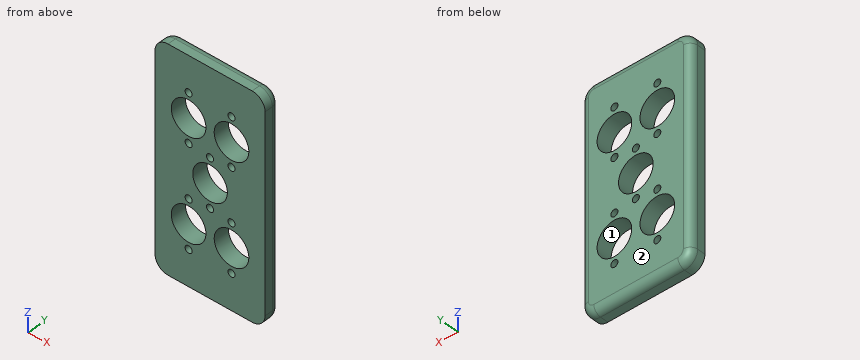
from build123d import *

# Parameters (mm, degrees)
SKETCH1_W             = 50.8
SKETCH1_H             = 101.6
BOSS_EXTRUDE1_DEPTH   = 7.25
FILLET1_R             = 6
FILLET2_R             = 3.5
CUT_EXTRUDE1_REACH    = 59.257
SKETCH2_R             = 8
F_4_CLEARANCE_HOLE1_D = 3.2639


with BuildPart() as part:
    # Sketch1 → Boss-Extrude1 (new body)
    with BuildSketch(Plane(origin=(0, 0, 0), x_dir=(1, 0, 0), z_dir=(0, 1, 0))):
        Rectangle(SKETCH1_W, SKETCH1_H)
    extrude(amount=BOSS_EXTRUDE1_DEPTH)

    # Fillet1
    fillet1_edges = [part.edges().sort_by_distance(p)[0] for p in [
        (25.4, 3.625, 50.8),
        (-25.4, 3.625, 50.8),
        (-25.4, 3.625, -50.8),
        (25.4, 3.625, -50.8),
    ]]
    fillet(fillet1_edges, radius=FILLET1_R)

    # Fillet2
    fillet2_edges = [part.edges().sort_by_distance(p)[0] for p in [
        (0, 7.25, -50.8),
        (25.4, 7.25, 0),
        (-25.4, 7.25, 0),
        (0, 7.25, 50.8),
        (23.642640687, 7.25, 49.042640687),
        (-23.642640687, 7.25, 49.042640687),
        (-23.642640687, 7.25, -49.042640687),
        (23.642640687, 7.25, -49.042640687),
    ]]
    fillet(fillet2_edges, radius=FILLET2_R)

    # Sketch2 → Cut-Extrude1 (cut, up to next)
    with BuildSketch(Plane.XZ, mode=Mode.PRIVATE) as cut_extrude1_sk1:
        with Locations(Location((0, 0, 0), (0, 0, 270))):
            Circle(SKETCH2_R)
    cut_extrude1_tool1 = extrude(cut_extrude1_sk1.sketch, amount=-CUT_EXTRUDE1_REACH, mode=Mode.PRIVATE) & part.part
    # Sketch2 → Cut-Extrude1 (cut, up to next)
    with BuildSketch(Plane.XZ, mode=Mode.PRIVATE) as cut_extrude1_sk2:
        with Locations(Location((9.9, 23.3, 0), (0, 0, 270))):
            Circle(SKETCH2_R)
    cut_extrude1_tool2 = extrude(cut_extrude1_sk2.sketch, amount=-CUT_EXTRUDE1_REACH, mode=Mode.PRIVATE) & part.part
    # Sketch2 → Cut-Extrude1 (cut, up to next)
    with BuildSketch(Plane.XZ, mode=Mode.PRIVATE) as cut_extrude1_sk3:
        with Locations(Location((-9.9, 23.3, 0), (0, 0, 270))):
            Circle(SKETCH2_R)
    cut_extrude1_tool3 = extrude(cut_extrude1_sk3.sketch, amount=-CUT_EXTRUDE1_REACH, mode=Mode.PRIVATE) & part.part
    # Sketch2 → Cut-Extrude1 (cut, up to next)
    with BuildSketch(Plane.XZ, mode=Mode.PRIVATE) as cut_extrude1_sk4:
        with Locations(Location((9.9, -23.3, 0), (0, 0, 270))):
            Circle(SKETCH2_R)
    cut_extrude1_tool4 = extrude(cut_extrude1_sk4.sketch, amount=-CUT_EXTRUDE1_REACH, mode=Mode.PRIVATE) & part.part
    # Sketch2 → Cut-Extrude1 (cut, up to next)
    with BuildSketch(Plane.XZ, mode=Mode.PRIVATE) as cut_extrude1_sk5:
        with Locations(Location((-9.9, -23.3, 0), (0, 0, 270))):
            Circle(SKETCH2_R)
    cut_extrude1_tool5 = extrude(cut_extrude1_sk5.sketch, amount=-CUT_EXTRUDE1_REACH, mode=Mode.PRIVATE) & part.part
    add(cut_extrude1_tool1.solids().sort_by_distance((0, 0, 0))[0], mode=Mode.SUBTRACT)
    add(cut_extrude1_tool2.solids().sort_by_distance((9.9, 0, 23.3))[0], mode=Mode.SUBTRACT)
    add(cut_extrude1_tool3.solids().sort_by_distance((-9.9, 0, 23.3))[0], mode=Mode.SUBTRACT)
    add(cut_extrude1_tool4.solids().sort_by_distance((9.9, 0, -23.3))[0], mode=Mode.SUBTRACT)
    add(cut_extrude1_tool5.solids().sort_by_distance((-9.9, 0, -23.3))[0], mode=Mode.SUBTRACT)

    # #4 Clearance Hole1 (through all)
    with Locations(Plane(origin=(0, 7.25, 0), x_dir=(-1, 0, 0), z_dir=(0, 1, 0))):
        with Locations((-9.9, 12.2), (-9.9, 34.4), (9.9, 34.4), (9.9, 12.2), (0, 11.1), (0, -11.1), (9.9, -12.2), (-9.9, -12.2), (9.9, -34.4), (-9.9, -34.4)):
            Hole(F_4_CLEARANCE_HOLE1_D / 2)


solid = part.part
Work out the finished part from the listing and answer in its coordinate system (mm). Face numbers are marked on the shaded views. Coordinates: 2 decimals unless noted, no trailing zeros. Loops run counter-clockwise (first coordinate to the right, second up) from the corner with the lowest first, then second, coordinate; pieces in that order, holes last. Notation, with made-up numbers: M 19.25,-0.75 L 76.25,-0.75 A26 cw 76.25,32.25 Z; hole C 17,2.25 d4. An arc over 180 degrees is marked long. Answer in a Markdown table with one row per item. Add a question column.
1. Flat-ended cylindrical pins translate along their axes: P1, Ø8, axis at x = 3.5, z = 13.5, coming from the -Y side; P2, Ø9.5, axis at x = 9.9, z = 23.3, coming from the -Y side; P3, Ø2, axis at y = 5, z = 4.5, coming from the -X side; P4, Ø3, axis at x = -16.5, y = 6, coming from the -Z side. Find the tip coordinate at first contact, or state that the pin passes through.
2. Consider L1, parallel to X at y = 1.5, z = -23; L2, parallel to X at y = 4.75, z = -23.3; L3, parallel to Z at x = 6.5, y = 5.5. Determine where each line is inside the solid, lowest interval first.
3. Find section B-B, the plane x = 9.9. State how many separate pieces and enclosed holes the cut face has, then the cut area to 3 significant figures.
4. Find section A-A, the plane z = 34.4. Write down the section's boundary in (x, y).
5. Find section D-D, the plane z = 5. Write down the section's boundary in (x, y) (3 decimals).
6. The mould has two halves that part along X. Classify the marked faces 1 and 2: pulls with the +X half, pulls with the -X half, needs draft (parallel to the pull), parting line crosses it, or undercut.
Reported:
| question | item | result |
|---|---|---|
| 1 | P1 | stops at y = 0 |
| 1 | P2 | passes through |
| 1 | P3 | stops at x = -25.39 |
| 1 | P4 | stops at z = -50.72 |
| 2 | L1 | x = -25.4 to -17.89, -1.91 to 1.91, 17.89 to 25.4 |
| 2 | L2 | x = -25.25 to -17.9, -1.9 to 1.9, 17.9 to 25.25 |
| 2 | L3 | z = -50.33 to -30.54, -16.06 to -4.66, 4.66 to 16.06, 30.54 to 50.33 |
| 3 | separate pieces | 7 |
| 3 | enclosed holes | 0 |
| 3 | area | 405 mm^2 |
| 4 | outline | M -25.4,0 L -11.53,0 L -11.53,7.25 L -21.9,7.25 A3.5 ccw -25.4,3.75 Z; M -8.27,0 L 8.27,0 L 8.27,7.25 L -8.27,7.25 Z; M 11.53,0 L 25.4,0 L 25.4,3.75 A3.5 ccw 21.9,7.25 L 11.53,7.25 Z |
| 5 | outline | M -25.4,0 L -6.245,0 L -6.245,7.25 L -21.9,7.25 A3.5 ccw -25.4,3.75 Z; M 6.245,0 L 25.4,0 L 25.4,3.75 A3.5 ccw 21.9,7.25 L 6.245,7.25 Z |
| 6 | face 1 | undercut |
| 6 | face 2 | needs draft |
